Here's how the part is built. I have some questions about the finished solid (model axes, mm). A direction names the side the tool comes from. Round coordinates to 2 decimals unless told otherwise and drop trailing zeros. Write each loop counter-clockwise with the first axis right and the second up, starting at its lowest first coordinate (ties: lowest second). Pieces come first, ordered by that corner, then holes. Notation, with made-up numbers: (-22, 60.25) -> (6, 60.25) arc R21 cw to (6, 74.25) -> close; hole circle Ø3 at (24, -40). An arc over 180 degrees is marked (long way). Put each result on its own line as item: value. Start each with the question number.
1) I want a section at A-A, the plane y = 8.75. List the corners of the cut face in (x, z) for me, then the cut area to 3 significant figures.
2) Will these pins go through, and if not, where does the flat tip stop? P1, Ø5, axis at x = -4, y = 5, coming from the -Z side; P2, Ø1, axis at x = -8.5, z = -4.5, coming from the +Y side; P3, Ø1, axis at x = 5.5, z = 5, coming from the +Y side.
3) Which directions (+Z, -Z, +X, -X, +Y, -Y) give clear straight access to the entire face, cutting with the end or side of a thin tool? Please do faces 1 (the flat face through (6.781, 7.528, -3.843)), 2 (the cylindrical face through (10, 2, 0)), 3 (the flat face through (6.72, 7.53, 3.95)), 4 (the flat face through (-6.72, 7.53, -3.95)), 5 (the flat face through (-3.8, 3.5, 7.5)).
4) If I drill on line 1 along Z through (x, y) = (0, 10.75); line 2 along Y through (x, z) = (-1.5, 9.5); line 3 along Z through (x, y) = (0, 8.25), over which ranges is the centre line in solid material (lowest first)? Write a range as [from, to].
from build123d import *

# Parameters (mm, degrees)
BOSS_EXTRUDE1_DEPTH = 4
SKETCH3_R           = 4.25
CUT_EXTRUDE1_DEPTH  = 10
CUT_EXTRUDE2_START  = -10
SKETCH4_R           = 4.25
CUT_EXTRUDE2_DEPTH  = 10
SKETCH5_OUTSIDE_W   = 33.422
SKETCH5_OUTSIDE_H   = 33.422
SKETCH5_OUTSIDE_R   = 8.25
CUT_EXTRUDE3_DEPTH  = 0.5
CHAMFER1_SIZE       = 1


# Read off the part's stored shape, not the designer's step: Cut-Extrude4
with BuildPart() as part:
    # Sketch1 → Revolve1 (revolve)
    with BuildSketch(Plane.XY, mode=Mode.PRIVATE) as revolve1_sk:
        Polygon((0, 0), (10, 0), (10, 4), (12, 4), (12, 6), (6, 6), (6, 15), (0, 15), align=None)
    revolve(revolve1_sk.sketch.rotate(Axis((0, 15, 0), (0, -1, 0)), 180), axis=Axis((0, 15, 0), (0, -1, 0)))

    # Sketch2 → Boss-Extrude1 (add)
    with BuildSketch(Plane(origin=(0, 6, 0), x_dir=(1, 0, 0), z_dir=(0, 1, 0))):
        Polygon((9, 0), (4.5, 7.794228634), (-4.5, 7.794228634), (-9, 0), (-4.5, -7.794228634), (4.5, -7.794228634), align=None)
    extrude(amount=BOSS_EXTRUDE1_DEPTH)

    # Sketch3 → Cut-Extrude1 (cut)
    with BuildSketch(Plane(origin=(0, 15, 0), x_dir=(1, 0, 0), z_dir=(0, 1, 0))):
        with Locations(Location((0, 0, 0), (0, 0, 180))):
            Circle(SKETCH3_R)
    extrude(amount=-CUT_EXTRUDE1_DEPTH, mode=Mode.SUBTRACT)

    # Sketch4 → Cut-Extrude2 (cut)
    with BuildSketch(Plane.XZ.offset(CUT_EXTRUDE2_START)):
        with Locations(Location((0, 0, 0), (0, 0, 180))):
            Circle(SKETCH4_R)
    extrude(amount=CUT_EXTRUDE2_DEPTH, mode=Mode.SUBTRACT)

    # Sketch5 outside → Cut-Extrude3 (cut)
    with BuildSketch(Plane.XZ.offset(-4)):
        Rectangle(SKETCH5_OUTSIDE_W, SKETCH5_OUTSIDE_H)
        Circle(SKETCH5_OUTSIDE_R, mode=Mode.SUBTRACT)
    extrude(amount=CUT_EXTRUDE3_DEPTH, mode=Mode.SUBTRACT)

    # Cut-Extrude4 outline → Cut-Extrude4 (revolve, cut)
    with BuildSketch(Plane.XY):
        Polygon((9.000000004, 10.000001017), (7.794228286, 10.000001017), (9.000000004, 7.911542725), align=None)
    revolve(axis=Axis((0, 0, 0), (0, 1, 0)), mode=Mode.SUBTRACT)

    # Chamfer1
    chamfer1_edges = [part.edges().sort_by_distance(p)[0] for p in [
        (4.25, 15, 0),
    ]]
    chamfer(chamfer1_edges, length=CHAMFER1_SIZE)


solid = part.part
Findings:
1. outline: (-8.47, -0.93) -> (-5.03, -6.87) arc R8.52 ccw to (-3.43, -7.79) -> (3.43, -7.79) arc R8.52 ccw to (5.03, -6.87) -> (8.47, -0.93) arc R8.52 ccw to (8.47, 0.93) -> (5.03, 6.87) arc R8.52 ccw to (3.43, 7.79) -> (-3.43, 7.79) arc R8.52 ccw to (-5.03, 6.87) -> (-8.47, 0.93) arc R8.52 ccw to start; hole circle Ø8.5 at (0, 0)
1. area: 151 mm2
2. P1: stops at z = -11.91
2. P2: stops at y = 6
2. P3: stops at y = 10
3. face 1: -Z, +X, +Y
3. face 2: -Y
3. face 3: +Z, +X, +Y
3. face 4: -Z, -X, +Y
3. face 5: none
4. line 1: z = [-6, -4.25], [4.25, 6]
4. line 2: y = [0, 3.5], [4, 6]
4. line 3: z = [-7.79, -4.25], [4.25, 7.79]
